Geometry check sheet. Reference: the model listing, model coordinates, mm. A direction names the side the tool comes from. Coordinates: 2 decimals unless noted, no trailing zeros. Loops run counter-clockwise (first coordinate to the right, second up) from the corner with the lowest first, then second, coordinate; pieces in that order, holes last. Notation, with made-up numbers: (46, 50) - (83, 50) arc R10 ccw to (83, 68) - close; hole circle Ø4 at (66.25, -33). An arc over 180 degrees is marked (long way). Write each question's results on one line, items separated by ' | '. Start each with the question number.
(1) Material ranges on probe 1 along Y at (x, z) = (0, -0.5); probe 2 along Z at (x, y) = (4.75, -9.5); probe 3 along Y at (x, z) = (-4.75, 5.5), recorded low to high.
(2) Access from +Z, -Z, +X, -X, +Y, -Y to the whole of each face (thin tool, end or side, straight path). Record for faces 4 (the face through (-1.67, 8.14, 4.762)), 5 (the face through (5, -5, 6.35)).
(3) Mould release check, pull along Y, two halves, no side actions. Record for faces 1 (the face through (-3, -6, -6.35)), 2 (the face through (10.6, 3.34, 5.56)), 3 (the face through (-0.83, 6.31, 0.09)): pulls with the +Y half, pulls with the -Y half, needs draft (parallel to the pull), parting line crosses it, or undercut.
(4) Sectioned sample at A-A (x = 0). Enter the section's corners in (y, z).
(5) Sectioned sample at C-C (z = -2.5). Enter the section's corners in (x, y).
(6) Go/stop test with flat-tipped pins: pin 1 Ø1 at (x, z) = (7, -2) entering from +Y; pin 2 Ø2 at (y, z) = (4.5, 5) entering from -X; pin 3 Ø1.5 at (x, z) = (-2.5, 0.5) entering from +Y. Record where each tip stops, or that it passes through.
from build123d import *

# Parameters (mm, degrees)
BOSS_EXTRUDE1_START = 6.35
SKETCH3_R           = 11.1125
SKETCH3_R_2         = 6.3627
BOSS_EXTRUDE1_DEPTH = 1.5875
BOSS_EXTRUDE2_START = 4.7625
SKETCH4_R           = 7.9502
SKETCH4_R_2         = 6.3627
BOSS_EXTRUDE2_DEPTH = 11.1125
CHAMFER1_SIZE       = 0.190881


with BuildPart() as part:
    # Sketch3 → Boss-Extrude1 (new body)
    with BuildSketch(Plane.XY.offset(BOSS_EXTRUDE1_START)):
        Circle(SKETCH3_R)
        Circle(SKETCH3_R_2, mode=Mode.SUBTRACT)
    extrude(amount=-BOSS_EXTRUDE1_DEPTH)

    # Sketch4 → Boss-Extrude2 (add)
    with BuildSketch(Plane.XY.offset(BOSS_EXTRUDE2_START)):
        Circle(SKETCH4_R)
        Circle(SKETCH4_R_2, mode=Mode.SUBTRACT)
    extrude(amount=-BOSS_EXTRUDE2_DEPTH)

    # Chamfer1
    chamfer1_edges = [part.edges().sort_by_distance(p)[0] for p in [
        (-6.3627, 0, -6.35),
        (-7.9502, 0, 4.7625),
        (-11.1125, 0, 6.35),
        (-11.1125, 0, 4.7625),
        (-6.3627, 0, 6.35),
        (-7.9502, 0, -6.35),
    ]]
    chamfer(chamfer1_edges, length=CHAMFER1_SIZE)


solid = part.part
Outcome:
1) probe 1: y = -7.95 to -6.36, 6.36 to 7.95 | probe 2: z = 4.76 to 6.35 | probe 3: y = -10.05 to -4.23, 4.23 to 10.05
2) face 4: -Z | face 5: +Z, +X, -X, +Y, -Y
3) face 1: needs draft | face 2: parting line crosses it | face 3: undercut
4) outline: (-11.11, 4.95) - (-10.92, 4.76) - (-8.14, 4.76) - (-7.95, 4.57) - (-7.95, -6.16) - (-7.76, -6.35) - (-6.55, -6.35) - (-6.36, -6.16) - (-6.36, 6.16) - (-6.55, 6.35) - (-10.92, 6.35) - (-11.11, 6.16) - close; (6.36, -6.16) - (6.55, -6.35) - (7.76, -6.35) - (7.95, -6.16) - (7.95, 4.57) - (8.14, 4.76) - (10.92, 4.76) - (11.11, 4.95) - (11.11, 6.16) - (10.92, 6.35) - (6.55, 6.35) - (6.36, 6.16) - close
5) outline: circle Ø15.9 at (0, 0); hole circle Ø12.73 at (0, 0)
6) pin 1: stops at y = 4.58 | pin 2: stops at x = -10.55 | pin 3: stops at y = 7.76
